```python
from build123d import *

# Parameters (mm, degrees)
ESBO_O1_W                   = 30
ESBO_O1_H                   = 50
ESBO_O1_W_2                 = 27
ESBO_O1_H_2                 = 47
RESSALTO_EXTRUS_O1_DEPTH    = 175
FURO_COM_FOLGA_DE_M53_D     = 5.5
FURO_COM_FOLGA_DE_M53_DEPTH = 30
FURO_COM_FOLGA_DE_M53_TIP   = 1.652366702
FURO_COM_FOLGA_DE_M85_D     = 9
FURO_COM_FOLGA_DE_M85_DEPTH = 30
FURO_COM_FOLGA_DE_M85_TIP   = 2.703872786


with BuildPart() as part:
    # Esboço1 → Ressalto-extrusão1 (new body)
    with BuildSketch(Plane.XY):
        with Locations((15, 25)):
            Rectangle(ESBO_O1_W, ESBO_O1_H)
        with Locations((15, 25)):
            Rectangle(ESBO_O1_W_2, ESBO_O1_H_2, mode=Mode.SUBTRACT)
    extrude(amount=RESSALTO_EXTRUS_O1_DEPTH)

    # Furo com folga de M53
    with Locations(Plane(origin=(30, 0, 0), x_dir=(0, 0, -1), z_dir=(1, 0, 0))):
        with Locations((-160, 43.5), (-160, 6.5)):
            Hole(FURO_COM_FOLGA_DE_M53_D / 2, depth=FURO_COM_FOLGA_DE_M53_DEPTH)
            with Locations((0, 0, -(FURO_COM_FOLGA_DE_M53_DEPTH + FURO_COM_FOLGA_DE_M53_TIP / 2))):  # 118° drill point
                Cone(0, FURO_COM_FOLGA_DE_M53_D / 2, FURO_COM_FOLGA_DE_M53_TIP, mode=Mode.SUBTRACT)

    # Furo com folga de M85
    with Locations(Plane(origin=(30, 0, 0), x_dir=(0, 0, -1), z_dir=(1, 0, 0))):
        with Locations((-160, 25)):
            Hole(FURO_COM_FOLGA_DE_M85_D / 2, depth=FURO_COM_FOLGA_DE_M85_DEPTH)
            with Locations((0, 0, -(FURO_COM_FOLGA_DE_M85_DEPTH + FURO_COM_FOLGA_DE_M85_TIP / 2))):  # 118° drill point
                Cone(0, FURO_COM_FOLGA_DE_M85_D / 2, FURO_COM_FOLGA_DE_M85_TIP, mode=Mode.SUBTRACT)


solid = part.part
```
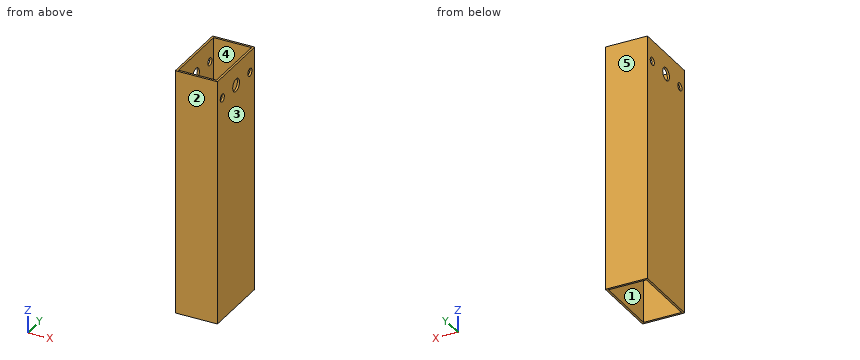
CAD build for the part. Positions are in the model's coordinates, mm. Face numbers are marked on the shaded views. A direction names the side the tool comes from. Coordinates: 2 decimals unless noted, no trailing zeros. Write each loop counter-clockwise with the first axis right and the second up, starting at its lowest first coordinate (ties: lowest second). Pieces come first, ordered by that corner, then holes. Notation, with made-up numbers: (13, 62.5) -> (32, 62.5) arc R11 cw to (32, 71.5) -> close; hole circle Ø6 at (1, -4). An arc over 180 degrees is marked (long way). Use CSV: the item, a comma, the result in double quotes. Start each with the question number.
Item 1: Two-plate mould, pull along X, no slides. Class the marked faces 3, 4 and 5: +X half, -X half, draft (parallel to the pull), parting line (faces both ways), or undercut.
Item 2: Wall check: probe 1 along Y at (x, z) = (0.8, 160); probe 2 along Y at (x, z) = (9.75, 122); probe 3 along X at (y, z) = (48, 134). Give the ranges that are in metal, low to high.
Item 3: Band-saw the part on A-A, the plane x = 13.5. Write the cut outline in (y, z), plus the area to 3 significant figures.
Item 4: Band-saw the part on D-D, the plane z = 109. Write the cut outline in (x, y).
Item 5: Band-saw the part on B-B, the plane z = 160. Give the number of separate pieces and of enclosed holes in the cut face, plus the area to 3 significant figures.
Item 6: Tool access for the marked faces 1 and 2: list every direction of +Z, -Z, +X, -X, +Y, -Y with a clear straight run to the whole face (end or side of a thin tool).
Item 7: Band-saw the part on C-C, the plane y = 6.5. Write the cut outline in (x, z).
Response values:
1,face 3,"+X half"
1,face 4,"undercut"
1,face 5,"draft"
2,probe 1,"y = 0 to 3.75, 9.25 to 20.5, 29.5 to 40.75, 46.25 to 50"
2,probe 2,"y = 0 to 1.5, 48.5 to 50"
2,probe 3,"x = 0 to 1.5, 28.5 to 30"
3,outline,"(0, 0) -> (1.5, 0) -> (1.5, 175) -> (0, 175) -> close; (48.5, 0) -> (50, 0) -> (50, 175) -> (48.5, 175) -> close"
3,area,"525 mm2"
4,outline,"(0, 0) -> (30, 0) -> (30, 50) -> (0, 50) -> close; hole (1.5, 1.5) -> (28.5, 1.5) -> (28.5, 48.5) -> (1.5, 48.5) -> close"
5,separate pieces,"6"
5,enclosed holes,"0"
5,area,"171 mm2"
6,face 1,"+Z, -Z"
6,face 2,"+Z, -Z, +X, -X, -Y"
7,outline,"(0, 0) -> (1.5, 0) -> (1.5, 157.25) -> (0, 157.25) -> close; (0, 162.75) -> (1.5, 162.75) -> (1.5, 175) -> (0, 175) -> close; (28.5, 0) -> (30, 0) -> (30, 157.25) -> (28.5, 157.25) -> close; (28.5, 162.75) -> (30, 162.75) -> (30, 175) -> (28.5, 175) -> close"
